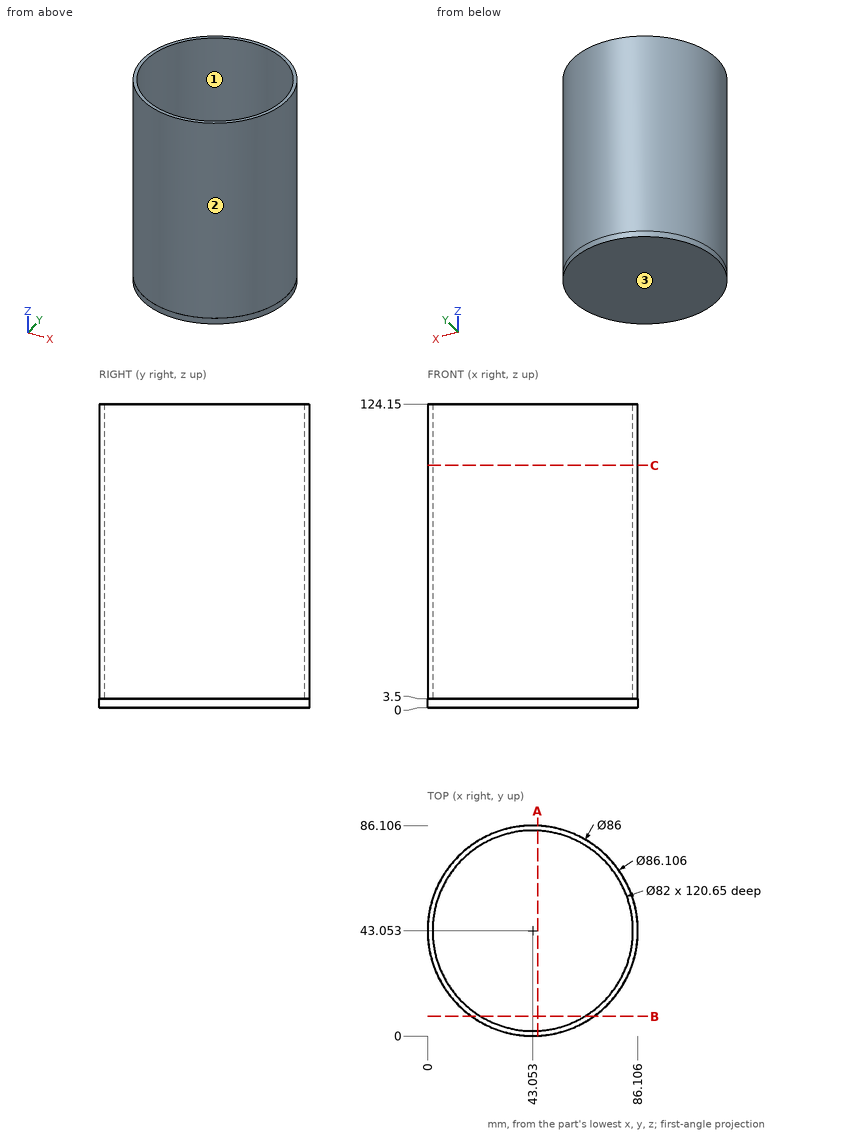
The figure shows three views and two pictorial views of one solid part (mm, origin at its lowest corner). Answer the questions. Round coordinates to 2 decimals unless told otherwise and drop trailing zeros. Write each loop counter-clockwise with the first axis right and the second up, starting at its lowest first coordinate (ties: lowest second). Pieces come first, ordered by that corner, then holes. Notation, with made-up numbers: (79.5, 32.5) - (116.5, 32.5) arc R28 ccw to (116.5, 52.5) - close; hole circle Ø3 at (18.25, 42). An arc over 180 degrees is marked (long way). Answer in a Markdown table with one row per item. Add a question column.
1. A cutting plane is placed at A-A, the plane x = 45. Determine the outline of the cut face in (y, z), and give its area (3 significant figures).
2. Given pin 1 (8 mm diameter, centred on y = 40.5, z = 106, fed in from +X); pin 2 (2 mm diameter, centred on x = 62, z = 60.5, fed in from -Y); pin 3 (2 mm diameter, centred on x = 41.5, z = 86, fed in from +Y), each flat-ended and moving along its own axis, determine where each tip first touches the part or whether it passes through.
3. A cutting plane is placed at B-B, the plane y = 8. Determine the outline of the cut face in (x, z), and give its area (3 significant figures).
4. The mould has two halves that part along Y. Classify the marked faces 1, 2 and 3: +Y half, -Y half, draft (parallel to the pull), parting line (faces both ways), or undercut.
5. Find the intervals of material crossed by line 1 along X through (y, z) = (42, 107.5); line 2 along Y through (x, z) = (44.5, 31.5); line 3 along Z through (x, y) = (78, 26.5), in increasing order. Write a range as from..to.
6. A cutting plane is placed at C-C, the plane z = 99. Determine the outline of the cut face in (x, y).
Worked out:
| question | item | result |
|---|---|---|
| 1 | outline | (0.04, 0) - (86.06, 0) - (86.06, 3.5) - (86.01, 3.5) - (86.01, 124.15) - (84.01, 124.15) - (84.01, 3.5) - (2.1, 3.5) - (2.1, 124.15) - (0.1, 124.15) - (0.1, 3.5) - (0.04, 3.5) - close |
| 1 | area | 784 mm^2 |
| 2 | pin 1 | x = 86.05 |
| 2 | pin 2 | y = 3.98 |
| 2 | pin 3 | y = 86.05 |
| 3 | outline | (18.06, 0) - (68.05, 0) - (68.05, 3.5) - (67.96, 3.5) - (67.96, 124.15) - (64.32, 124.15) - (64.32, 3.5) - (21.79, 3.5) - (21.79, 124.15) - (18.15, 124.15) - (18.15, 3.5) - (18.06, 3.5) - close |
| 3 | area | 1,050 mm^2 |
| 4 | face 1 | undercut |
| 4 | face 2 | parting line |
| 4 | face 3 | draft |
| 5 | line 1 | 0.07..2.07, 84.04..86.04 |
| 5 | line 2 | 0.08..2.08, 84.03..86.03 |
| 5 | line 3 | 0..3.5 |
| 6 | outline | circle Ø86 at (43.05, 43.05); hole circle Ø82 at (43.05, 43.05) |
